The figure shows three views and two pictorial views of one solid part (mm, origin at its lowest corner). Answer the questions. Coordinates: 2 decimals unless noted, no trailing zeros. Loops run counter-clockwise (first coordinate to the right, second up) from the corner with the lowest first, then second, coordinate; pieces in that order, holes last. Notation, with made-up numbers: (78, 60) - (96, 60) arc R16 cw to (96, 82) - close; hole circle Ø9 at (38.25, 14). An arc over 180 degrees is marked (long way). Return JSON: item names as keys, results as strings. Group by question number.
1. The mould has two halves that part along Y. Classify the marked faces 1, 2 and 3: pulls with the +Y half, pulls with the -Y half, needs draft (parallel to the pull), parting line crosses it, or undercut.
2. Each of these flat-tipped pins is pushed along its axis until it touches: P1, Ø1.6, axis at y = 8.5, z = 2.5, coming from the -X side; P2, Ø3.5, axis at x = 2.8, y = 2.8, coming from the +Z side; P3, Ø8, axis at x = 10.5, y = 4, coming from the -Z side; P4, Ø1.6, axis at y = 7.5, z = 2.5, coming from the +X side. Where does it stop, or does it pass through?
3. Find the intervals of material crossed by line 1 along Y through (x, z) = (2.8, 1.3); line 2 along X through (y, z) = (1.75, 0.3); line 3 along X through (y, z) = (3.5, 0.6), in increasing order.
4. Section A-A (x = 2.8) is taken. Write down the section's boundary in (y, z), and give its area (3 significant figures).
5. Section C-C (z = 0.4) is taken. Write down the section's boundary in (x, y).
6. Section B-B (y = 2.8) is taken. Write down the section's boundary in (x, z), and give its area (3 significant figures).
7. Section D-D (x = 8.5) is taken. Write down the section's boundary in (y, z), and give its area (3 significant figures).
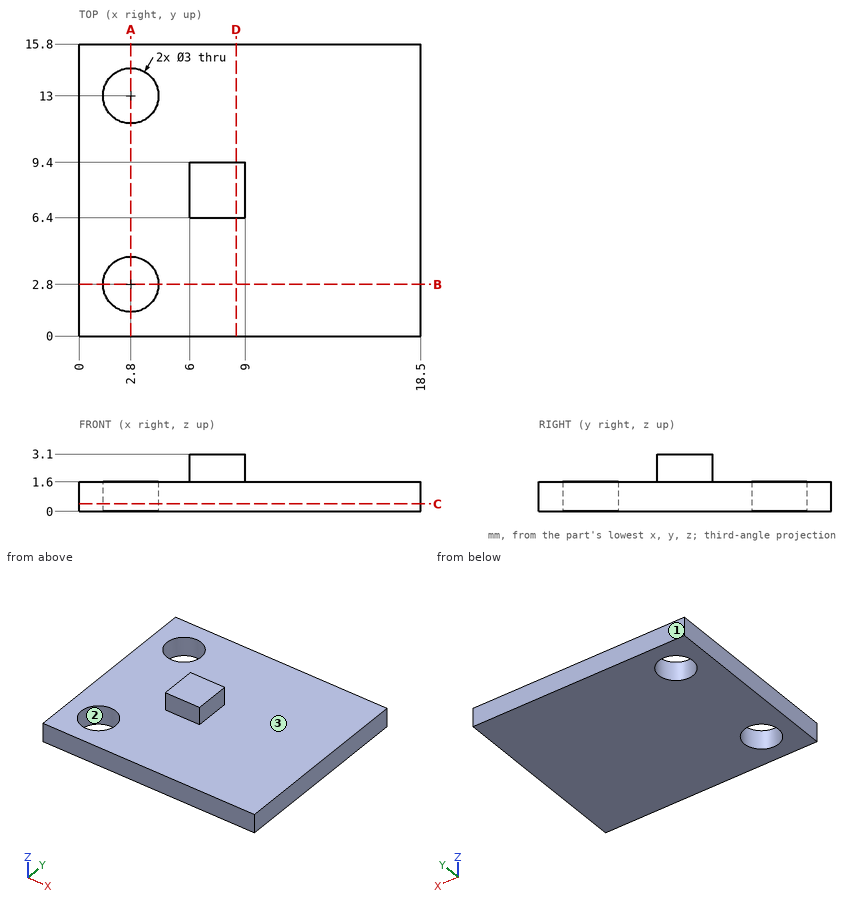
The answers:
{
 "1": {"face 1": "pulls with the +Y half", "face 2": "undercut", "face 3": "needs draft"},
 "2": {"P1": "stops at x = 6", "P2": "stops at z = 1.6", "P3": "stops at z = 0", "P4": "stops at x = 9"},
 "3": {"line 1": "y = 0 to 1.3, 4.3 to 11.5, 14.5 to 15.8", "line 2": "x = 0 to 1.73, 3.87 to 18.5", "line 3": "x = 0 to 1.47, 4.13 to 18.5"},
 "4": {"outline": "(0, 0) - (1.3, 0) - (1.3, 1.6) - (0, 1.6) - close; (4.3, 0) - (11.5, 0) - (11.5, 1.6) - (4.3, 1.6) - close; (14.5, 0) - (15.8, 0) - (15.8, 1.6) - (14.5, 1.6) - close", "area": "15.7 mm2"},
 "5": {"outline": "(0, 0) - (18.5, 0) - (18.5, 15.8) - (0, 15.8) - close; hole circle Ø3 at (2.8, 2.8); hole circle Ø3 at (2.8, 13)"},
 "6": {"outline": "(0, 0) - (1.3, 0) - (1.3, 1.6) - (0, 1.6) - close; (4.3, 0) - (18.5, 0) - (18.5, 1.6) - (4.3, 1.6) - close", "area": "24.8 mm2"},
 "7": {"outline": "(0, 0) - (15.8, 0) - (15.8, 1.6) - (9.4, 1.6) - (9.4, 3.1) - (6.4, 3.1) - (6.4, 1.6) - (0, 1.6) - close", "area": "29.8 mm2"}
}
